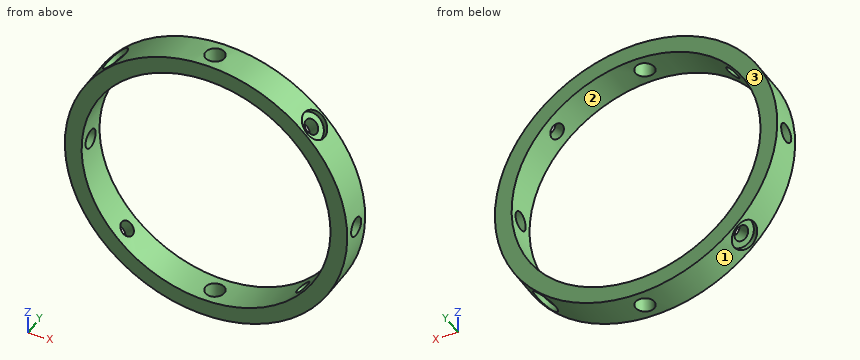
```python
from build123d import *

# Parameters (mm, degrees)
SKETCH1_R                = 29.5
SKETCH1_R_2              = 26
BOSS_EXTRUDE1_DEPTH      = 3.5
BOSS_EXTRUDE1_DEPTH_BACK = 3.5
SKETCH3_R                = 1.975
CUT_EXTRUDE1_DEPTH       = 42.865857211
CUT_EXTRUDE1_DEPTH_BACK  = 42.865857211
SKETCH4_R                = 1.975
CUT_EXTRUDE2_DEPTH       = 42.865857362
CUT_EXTRUDE2_DEPTH_BACK  = 42.865857362
SKETCH5_R                = 1.6
CUT_EXTRUDE3_DEPTH       = 42.865857364
CUT_EXTRUDE3_DEPTH_BACK  = 42.865857364
SKETCH6_R                = 1.6
CUT_EXTRUDE4_DEPTH       = 42.865857364
CUT_EXTRUDE4_DEPTH_BACK  = 42.865857364
CUT_EXTRUDE5_REACH       = 73.305
CUT_EXTRUDE5_END_RADIUS  = 28.5
SKETCH7_R                = 3
CIRPATTERN1_COUNT        = 4


with BuildPart() as part:
    # Sketch1 → Boss-Extrude1 (new, two sides)
    with BuildSketch(Plane(origin=(0, 0, 0), x_dir=(1, 0, 0), z_dir=(0, 1, 0))) as boss_extrude1_sk:
        with Locations(Location((0, 0, 0), (0, 0, 270))):
            Circle(SKETCH1_R)
        with Locations(Location((0, 0, 0), (0, 0, 270))):
            Circle(SKETCH1_R_2, mode=Mode.SUBTRACT)
    extrude(amount=BOSS_EXTRUDE1_DEPTH)
    extrude(boss_extrude1_sk.sketch, amount=-BOSS_EXTRUDE1_DEPTH_BACK)

    # Sketch3 → Cut-Extrude1 (cut, two sides)
    with BuildSketch(Plane(origin=(0, 0, 0), x_dir=(0, 0, -1), z_dir=(1, 0, 0))) as cut_extrude1_sk:
        Circle(SKETCH3_R)
    extrude(amount=CUT_EXTRUDE1_DEPTH, mode=Mode.SUBTRACT)
    extrude(cut_extrude1_sk.sketch, amount=-CUT_EXTRUDE1_DEPTH_BACK, mode=Mode.SUBTRACT)

    # Sketch4 → Cut-Extrude2 (cut, two sides)
    with BuildSketch(Plane.XY) as cut_extrude2_sk:
        Circle(SKETCH4_R)
    extrude(amount=CUT_EXTRUDE2_DEPTH, mode=Mode.SUBTRACT)
    extrude(cut_extrude2_sk.sketch, amount=-CUT_EXTRUDE2_DEPTH_BACK, mode=Mode.SUBTRACT)

    # Sketch5 → Cut-Extrude3 (cut, two sides)
    with BuildSketch(Plane(origin=(0, 0, 0), x_dir=(-0.7071067811865477, 0, -0.7071067811865475), z_dir=(0.7071067811865475, 0, -0.7071067811865477))) as cut_extrude3_sk:
        Circle(SKETCH5_R)
    extrude(amount=CUT_EXTRUDE3_DEPTH, mode=Mode.SUBTRACT)
    extrude(cut_extrude3_sk.sketch, amount=-CUT_EXTRUDE3_DEPTH_BACK, mode=Mode.SUBTRACT)

    # Sketch6 → Cut-Extrude4 (cut, two sides)
    with BuildSketch(Plane(origin=(0, 0, 0), x_dir=(0.7071067811865476, 0, -0.7071067811865476), z_dir=(0.7071067811865476, 0, 0.7071067811865476))) as cut_extrude4_sk:
        Circle(SKETCH6_R)
    extrude(amount=CUT_EXTRUDE4_DEPTH, mode=Mode.SUBTRACT)
    extrude(cut_extrude4_sk.sketch, amount=-CUT_EXTRUDE4_DEPTH_BACK, mode=Mode.SUBTRACT)

    # Cut-Extrude5: up to this cylinder (the profile starts outside it)
    cut_extrude5_end = Plane(origin=(0, 0, 0), z_dir=(0, 1, 0)) * Cylinder(CUT_EXTRUDE5_END_RADIUS, 204.61, mode=Mode.PRIVATE)
    # Sketch7 → Cut-Extrude5 (cut, up to the surface)
    with BuildSketch(Plane(origin=(20.859650045, 0, 20.859650045), x_dir=(0.7071067811865475, 0, -0.7071067811865477), z_dir=(0.7071067811865477, 0, 0.7071067811865475)), mode=Mode.PRIVATE) as cut_extrude5_sk1:
        Circle(SKETCH7_R)
    cut_extrude5_tool1 = extrude(cut_extrude5_sk1.sketch, amount=-CUT_EXTRUDE5_REACH, mode=Mode.PRIVATE) - cut_extrude5_end
    cut_extrude5 = cut_extrude5_tool1.solids().sort_by_distance((20.85965, 0, 20.85965))[0]
    add(cut_extrude5, mode=Mode.SUBTRACT)

    # CirPattern1: Cut-Extrude5 ×4 about axis
    cirpattern1_axis = Axis((0, 0, 0), (0, 1, 0))
    for i in range(1, CIRPATTERN1_COUNT):
        add(cut_extrude5.rotate(cirpattern1_axis, i * 360 / CIRPATTERN1_COUNT), mode=Mode.SUBTRACT)


solid = part.part
```
Geometry check sheet. Reference: the model listing, model coordinates, mm. Face numbers are marked on the shaded views. Coordinates: 2 decimals unless noted, no trailing zeros. Write each loop counter-clockwise with the first axis right and the second up, starting at its lowest first coordinate (ties: lowest second). Pieces come first, ordered by that corner, then holes. Notation, with made-up numbers: M -25.5,53 L -0.5,53 A6 cw -0.5,57 Z; hole C 2,34 d6. An arc over 180 degrees is marked long. Answer as a JSON object with one key per item and string values.
1. Section check B-B, the plane z = 0. Enter the section's corners in (x, y) (3 decimals).
Answers below:
{"outline": "M -29.5,-3.5 L -26,-3.5 L -26,-1.975 L -29.5,-1.975 Z; M -29.5,1.975 L -26,1.975 L -26,3.5 L -29.5,3.5 Z; M 26,-3.5 L 29.5,-3.5 L 29.5,-1.975 L 26,-1.975 Z; M 26,1.975 L 29.5,1.975 L 29.5,3.5 L 26,3.5 Z"}
2. Section check A-A, the plane x = 0. Enter the section's corners in (y, z) (3 decimals).
Answers below:
{"outline": "M -3.5,-29.5 L -1.975,-29.5 L -1.975,-26 L -3.5,-26 Z; M -3.5,26 L -1.975,26 L -1.975,29.5 L -3.5,29.5 Z; M 1.975,-29.5 L 3.5,-29.5 L 3.5,-26 L 1.975,-26 Z; M 1.975,26 L 3.5,26 L 3.5,29.5 L 1.975,29.5 Z"}
3. Scan lines: L1, parallel to Z at x = -0.5, y = -3; L2, parallel to Y at x = 28.35, z = 0 (3 decimals); L3, parallel to Z at x = -13, y = 1.5. Record each from-to range of solid material in increasing order.
Answers below:
{"L1": "z = -29.5 to -26, 26 to 29.5", "L2": "y = -3.5 to -1.975, 1.975 to 3.5", "L3": "z = -26.48 to -22.52, 22.52 to 26.48"}
4. Section check C-C, the plane z = -10. Enter the section's corners in (x, y).
Answers below:
{"outline": "M -27.75,-3.5 L -24,-3.5 L -24,3.5 L -27.75,3.5 Z; M 24,-3.5 L 27.75,-3.5 L 27.75,3.5 L 24,3.5 Z"}
5. Section check D-D, the plane y = 0. Give the number of separate pieces and of enclosed holes in the cut face, plus the area to 3 significant figures.
Answers below:
{"separate pieces": "8", "enclosed holes": "0", "area": "499 mm²"}
6. Draft check along Z on the marked faces 1, 2 and 3. Enter one of: released by +Z, released by -Z, zero draft, split by the parting line, or undercut.
Answers below:
{"face 1": "split by the parting line", "face 2": "undercut", "face 3": "zero draft"}
7. Go/stop test with flat-tipped pins: pin 1 Ø3 at (y, z) = (0.5, 17) entering from -X; pin 2 Ø1 at (y, z) = (-2.5, 2.5) entering from -X; pin 3 Ø1.5 at (y, z) = (1.5, 5.5) entering from -X; pin 4 Ø3 at (y, z) = (0, 0) entering from -X (3 decimals). Record where each tip stops, or that it passes through.
Answers below:
{"pin 1": "stops at x = -25.1", "pin 2": "stops at x = -29.43", "pin 3": "stops at x = -29.12", "pin 4": "passes through"}
